Part model, mm, in its own coordinate system. Face numbers are marked on the shaded views. A direction names the side the tool comes from. Coordinates: 2 decimals unless noted, no trailing zeros. Loops run counter-clockwise (first coordinate to the right, second up) from the corner with the lowest first, then second, coordinate; pieces in that order, holes last. Notation, with made-up numbers: (15.25, 24.5) - (36.25, 24.5) arc R9 cw to (36.25, 36.5) - close; hole circle Ø9 at (66.5, 12.5). An arc over 180 degrees is marked (long way). Answer as CSV lines item,"result".
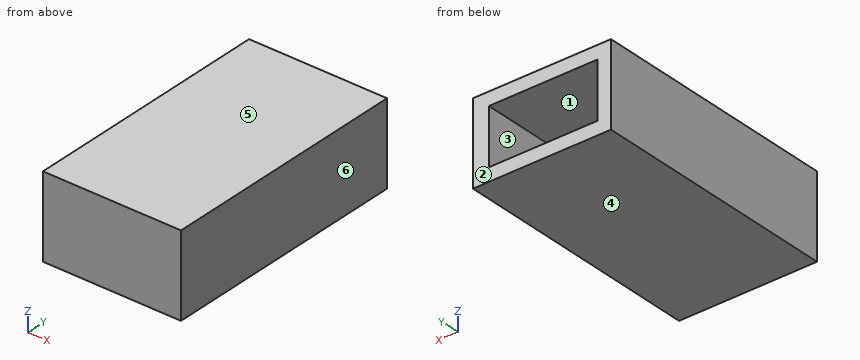
Autodesk Inventor part; units mm, degrees
ref_plane "YZ Plane" through (0, 0, 0) normal (1, 0, 0) x (0, 1, 0)
ref_plane "XZ Plane" through (0, 0, 0) normal (0, 1, 0) x (-1, 0, 0)
ref_plane "XY Plane" through (0, 0, 0) normal (0, 0, 1) x (1, 0, 0)
sketch "Sketch2" plane through (0, 0, 0) normal (0, 1, 0) x (-1, 0, 0)
  line L0 (-5.2, -3.1) -> (5.2, -3.1)
  line L1 (5.2, -3.1) -> (5.2, 3.1)
  line L2 (5.2, 3.1) -> (-5.2, 3.1)
  line L3 (-5.2, 3.1) -> (-5.2, -3.1)
  line L4 (-5.2, -3.1) -> (5.2, 3.1) construction
  line L5 (5.2, -3.1) -> (-5.2, 3.1) construction
  point P0 (0, 0)
  dimension "d10" = 10.4
  dimension "d11" = 6.2
extrude "Extrusion1" add sketch "Sketch2" along normal blind 14
sketch "Sketch3" plane through (0, 14, 0) normal (0, 1, 0) x (1, 0, 0)
  line L0 (5.2, 3.1) -> (-5.2, 3.1)
  line L1 (-5.2, 3.1) -> (-5.2, -3.1)
  line L2 (-4.2, 2.1) -> (4, 2.1)
  line L3 (4, 2.1) -> (4, 0.5)
  line L4 (4, 0.5) -> (-4.2, 0.5)
  line L5 (-4.2, 0.5) -> (-4.2, 2.1)
  point P0 (0, 0)
  dimension "d14" = 8.2
  dimension "d15" = 1.6
  dimension "d16" = 1
  dimension "d17" = 1
extrude "Extrusion2" cut sketch "Sketch3" against normal blind 0.5
sketch "Sketch4" plane through (0, 14, 0) normal (0, 1, 0) x (1, 0, 0)
  line L0 (-4.2, 2.1) -> (4, 2.1)
  line L1 (-5.2, -3.1) -> (5.2, -3.1)
  line L2 (-4.2, 0.5) -> (4, 0.5)
  line L3 (4, 0.5) -> (4, -2.1)
  line L4 (4, -2.1) -> (-4.2, -2.1)
  line L5 (-4.2, -2.1) -> (-4.2, 0.5)
  point P0 (0, 0)
  dimension "d20" = 1
extrude "Extrusion3" cut sketch "Sketch4" against normal blind 12
sketch "Sketch5" plane through (0, 14, 0) normal (0, 1, 0) x (1, 0, 0)
  line L0 (-5.2, 3.1) -> (5.2, 3.1)
  line L1 (5.2, 3.1) -> (5.2, -3.1)
  line L2 (5.2, -3.1) -> (-5.2, -3.1)
  line L3 (-5.2, -3.1) -> (-5.2, 3.1)
  line L4 (4, -2.1) -> (-4.2, -2.1)
  line L5 (-4.2, -2.1) -> (-4.2, 2.1)
  line L6 (-4.2, 2.1) -> (4, 2.1)
  line L7 (4, 2.1) -> (4, -2.1)
  point P0 (0, 0)
extrude "Extrusion4" add sketch "Sketch5" along normal blind 5
properties part number "test"
Q1. Two-plate mould, pull along Z, no slides. Class the marked faces 3, 4, 5 and 6: released by +Z, released by -Z, zero draft, split by the parting line, or undercut.
Results:
face 3,"undercut"
face 4,"released by -Z"
face 5,"released by +Z"
face 6,"zero draft"
Q2. Wall check: L1, parallel to Z at x = 1.5, y = 12.25; L2, parallel to Z at x = 2.75, y = 17.5; L3, parallel to X at y = 7.5, z = 2. Give the ranges that are in metal, low to high.
Results:
L1,"z = -3.1 to -0.5, 2.1 to 3.1"
L2,"z = -3.1 to -2.1, 2.1 to 3.1"
L3,"x = -5.2 to -4.2, 4 to 5.2"
Q3. Saw through at D-D (y = 10). Give the cut face in (x, z), then the cut area to 3 significant figures.
Results:
outline,"(-5.2, -3.1) - (5.2, -3.1) - (5.2, 3.1) - (-5.2, 3.1) - close; hole (-4.2, -0.5) - (4, -0.5) - (4, 2.1) - (-4.2, 2.1) - close"
area,"43.2 mm^2"
Q4. Flat gauge pin, fed straight in: pin 1 (0.5 mm diameter, centred on x = -1.5, z = -1, fed in from +Y). Where does the tip first touch, or does it go through?
Results:
pin 1,"stops at y = 13.5"
Q5. Which spindle directions (+Z, -Z, +X, -X, +Y, -Y) get a long thin tool onto all of the face, cutting with end or side? Do the marked faces 1 and 2. Say none if no direction does.
Results:
face 1,"+Y"
face 2,"+Z, -Z, +X, -X, +Y"
Q6. Saw through at A-A (y = 15). Give the cut face in (x, z), then the cut area to 3 significant figures.
Results:
outline,"(-5.2, -3.1) - (5.2, -3.1) - (5.2, 3.1) - (-5.2, 3.1) - close; hole (-4.2, -2.1) - (4, -2.1) - (4, 2.1) - (-4.2, 2.1) - close"
area,"30.0 mm^2"
Q7. Saw through at B-B (z = 0.5). Give the cut face in (x, y).
Results:
outline,"(-5.2, 0) - (5.2, 0) - (5.2, 19) - (4, 19) - (4, 2) - (-4.2, 2) - (-4.2, 19) - (-5.2, 19) - close"
Q8. Saw through at C-C (x = 2.75). Give the cut face in (y, z), then the cut area to 3 significant figures.
Results:
outline,"(0, -3.1) - (19, -3.1) - (19, -2.1) - (13.5, -2.1) - (13.5, -0.5) - (2, -0.5) - (2, 2.1) - (19, 2.1) - (19, 3.1) - (0, 3.1) - close"
area,"64.8 mm^2"
